Here's how the part is built. I have some questions about the finished solid (model axes, mm). Round coordinates to 2 decimals unless told otherwise and drop trailing zeros. Order: outer loops, then holes, each group sorted by start corner. A loop starts at its lowest first (then second) coordinate and runs counter-clockwise, first axis right, second up. Notation, with made-up numbers: (-3.5, 56.25) -> (25.5, 56.25) arc R21 cw to (25.5, 65.25) -> close; hole circle Ø10 at (66.5, -9). An arc over 180 degrees is marked (long way). Use a Markdown table: item, result. Add a question column.
(1) I want a section at A-A, the plane z = -196. Please give me the cut outline in (x, y) (3 decimals).
(2) I'm going to push flat-ended pins straight in: P1, Ø4.5, axis at y = 4.63, z = -273.28, coming from the +X side; P2, Ø1.6, axis at x = 1, z = -390, coming from the -Y side; P3, Ø1, axis at x = 1.5, z = -354, coming from the -Y side; P4, Ø1, axis at x = 2.5, z = -388.5, coming from the +Y side. Where does each tip first touch, or does it pass through?
(3) If I drill on probe 1 along Z at (x, y) = (1.5, 31); probe 2 along Y at (x, z) = (0.85, -200.5); probe 3 along Y at (x, z) = (0.4, -272.5), over which ranges is the centre line in solid material (lowest first)?
(4) I want a section at C-C, the plane x = 2.25. Give the number of separate pieces and of enclosed holes in the cut face, then the cut area to 3 significant figures.
(5) I want a section at D-D, the plane y = 104.5. Please give me the cut outline in (x, z) (3 decimals), then the cut area to 3 significant figures.
(6) I want a section at B-B, the plane z = -59. Please give me the cut outline in (x, y) (3 decimals), then the cut area to 3 significant figures.
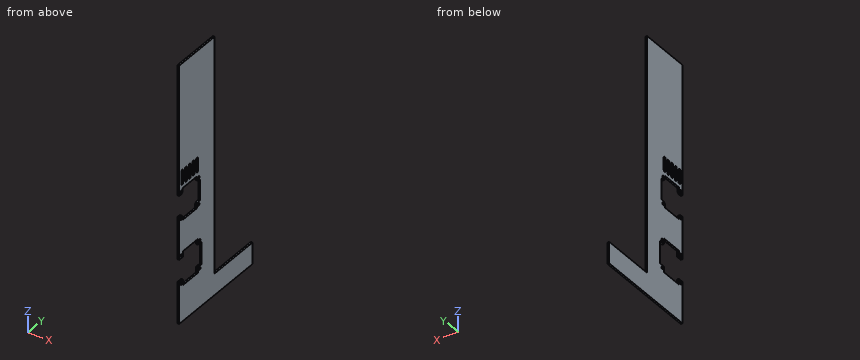
Autodesk Inventor part; units mm, degrees
ref_plane "YZ Plane" through (0, 0, 0) normal (1, 0, 0) x (0, 1, 0)
ref_plane "XZ Plane" through (0, 0, 0) normal (0, 1, 0) x (-1, 0, 0)
ref_plane "XY Plane" through (0, 0, 0) normal (0, 0, 1) x (1, 0, 0)
sketch "Sketch1" plane through (0, 0, 0) normal (1, 0, 0) x (0, 1, 0)
  line L0 (0, 0) -> (95.25, 0)
  line L1 (95.25, 0) -> (95.25, -419.1)
  line L2 (95.25, -457.2) -> (0, -457.2)
  line L3 (0, -457.2) -> (0, 0)
  line L4 (0, -457.2) -> (196.85, -457.2)
  line L5 (196.85, -457.2) -> (196.85, -419.1)
  line L6 (196.85, -419.1) -> (95.25, -419.1)
  line L7 (0, -419.1) -> (0, -457.2)
extrude "Extrusion1" add sketch "Sketch1" along normal blind 3.175
sketch "Sketch2" plane through (0, 0, 0) normal (-1, 0, 0) x (0, 0, 1)
  line L0 (-393.7, 49.9364) -> (-393.7, 10.0076)
  line L1 (-333.756, 10.0076) -> (-333.756, 49.9364)
  line L2 (-343.7636, 59.944) -> (-383.6924, 59.944)
  circle A0 centre (-388.6962, 54.9402) radius 2.159
  circle A1 centre (-338.7598, 54.9402) radius 2.159
  circle A2 centre (-388.6962, 5.0038) radius 2.159
  circle A3 centre (-338.7598, 5.0038) radius 2.159
  line L3 (-383.6924, 59.944) -> (-383.6924, 49.9364)
  line L4 (-383.6924, 49.9364) -> (-393.7, 49.9364)
  line L5 (-343.7636, 59.944) -> (-343.7636, 49.9364)
  line L6 (-343.7636, 49.9364) -> (-333.756, 49.9364)
  line L7 (-383.6924, 0) -> (-383.6924, 10.0076)
  line L8 (-383.6924, 10.0076) -> (-393.7, 10.0076)
  line L9 (-343.7636, 0) -> (-343.7636, 10.0076)
  line L10 (-343.7636, 10.0076) -> (-333.756, 10.0076)
  circle A4 centre (-273.2786, 51.7724) radius 2.54
  circle A5 centre (-273.2786, 4.63) radius 2.54
  circle A6 centre (-226.1362, 51.7724) radius 2.54
  circle A7 centre (-226.1362, 4.63) radius 2.54
  line L11 (-190.9572, 5.646) -> (-212.4456, 5.646)
  line L12 (-212.4456, 10.726) -> (-190.9572, 10.726)
  arc A8 (-190.9572, 5.646) -> (-190.9572, 10.726) centre (-190.9572, 8.186) ccw
  arc A9 (-212.4456, 10.726) -> (-212.4456, 5.646) centre (-212.4456, 8.186) ccw
  line L13 (-190.9572, 15.6282) -> (-212.4456, 15.6282)
  line L14 (-212.4456, 20.7082) -> (-190.9572, 20.7082)
  arc A10 (-190.9572, 15.6282) -> (-190.9572, 20.7082) centre (-190.9572, 18.1682) ccw
  arc A11 (-212.4456, 20.7082) -> (-212.4456, 15.6282) centre (-212.4456, 18.1682) ccw
  line L15 (-190.9572, 25.6104) -> (-212.4456, 25.6104)
  line L16 (-212.4456, 30.6904) -> (-190.9572, 30.6904)
  arc A12 (-190.9572, 25.6104) -> (-190.9572, 30.6904) centre (-190.9572, 28.1504) ccw
  arc A13 (-212.4456, 30.6904) -> (-212.4456, 25.6104) centre (-212.4456, 28.1504) ccw
  line L17 (-190.9572, 35.5926) -> (-212.4456, 35.5926)
  line L18 (-212.4456, 40.6726) -> (-190.9572, 40.6726)
  arc A14 (-190.9572, 35.5926) -> (-190.9572, 40.6726) centre (-190.9572, 38.1326) ccw
  arc A15 (-212.4456, 40.6726) -> (-212.4456, 35.5926) centre (-212.4456, 38.1326) ccw
  line L19 (-190.9572, 45.5748) -> (-212.4456, 45.5748)
  line L20 (-212.4456, 50.6548) -> (-190.9572, 50.6548)
  arc A16 (-190.9572, 45.5748) -> (-190.9572, 50.6548) centre (-190.9572, 48.1148) ccw
  arc A17 (-212.4456, 50.6548) -> (-212.4456, 45.5748) centre (-212.4456, 48.1148) ccw
  line L21 (-457.2, 0) -> (-457.2, 196.85)
  line L22 (-457.2, 0) -> (-393.7, 0)
  line L23 (-383.6924, 0) -> (-343.7636, 0)
  line L24 (-419.1, 95.25) -> (0, 95.25)
  line L25 (-4.8028, 0) -> (-4.8028, 95.25)
  line L26 (-4.8028, 95.25) -> (-457.2, 95.25)
  line L27 (-457.2, 95.25) -> (-457.2, 0)
  line L28 (-267.3803, 56.4007) -> (-232.0345, 56.4007)
  line L29 (-221.5079, 45.8741) -> (-221.5079, 10.5283)
  line L30 (-232.0345, 0) -> (-267.3803, 0)
  line L31 (-277.9086, 10.5283) -> (-277.9086, 45.8741)
  line L32 (-273.2786, 51.7724) -> (-271.5234, 49.9364)
  line L33 (-271.5234, 49.9364) -> (-270.4878, 48.8532)
  arc A18 (-268.6503, 4.5045) -> (-273.4041, 9.2583) centre (-273.2786, 4.63) ccw
  arc A19 (-226.1362, 9.2583) -> (-230.7645, 4.63) centre (-226.1362, 4.63) ccw
  arc A20 (-230.7645, 51.7724) -> (-226.1362, 47.1441) centre (-226.1362, 51.7724) ccw
  arc A21 (-273.2786, 47.1441) -> (-268.6503, 51.7724) centre (-273.2786, 51.7724) ccw
  line L34 (-268.6503, 55.1307) -> (-268.6503, 51.7724)
  line L35 (-273.2786, 47.1441) -> (-276.6386, 47.1441)
  line L36 (-230.7645, 55.1307) -> (-230.7645, 51.7724)
  line L37 (-226.1362, 47.1441) -> (-222.7779, 47.1441)
  line L38 (-221.5079, 0) -> (-230.7645, 0)
  line L39 (-230.7645, 1.27) -> (-230.7645, 4.63)
  line L40 (-226.1362, 9.2583) -> (-222.7779, 9.2583)
  line L41 (-277.9086, 0) -> (-268.6503, 0)
  line L42 (-268.6503, 1.27) -> (-268.6503, 4.7555)
  line L43 (-273.1531, 9.2583) -> (-276.6386, 9.2583)
  arc A22 (-277.9086, 10.5283) -> (-276.6386, 9.2583) centre (-276.6386, 10.5283) ccw
  arc A23 (-267.3803, 56.4007) -> (-268.6503, 55.1307) centre (-267.3803, 55.1307) ccw
  arc A24 (-276.6386, 47.1441) -> (-277.9086, 45.8741) centre (-276.6386, 45.8741) ccw
  arc A25 (-230.7645, 55.1307) -> (-232.0345, 56.4007) centre (-232.0345, 55.1307) ccw
  arc A26 (-221.5079, 45.8741) -> (-222.7779, 47.1441) centre (-222.7779, 45.8741) ccw
  arc A27 (-222.7779, 9.2583) -> (-221.5079, 10.5283) centre (-222.7779, 10.5283) ccw
  line L44 (-277.9086, 56.4007) -> (-277.7032, 56.4007)
  line L45 (-268.6503, 4.5045) -> (-268.6503, 0)
  line L46 (0, 0) -> (-457.2, 0)
  line L47 (-230.7645, 4.63) -> (-230.7645, 0)
  line L48 (-268.6503, 0) -> (-230.7645, 0)
  dimension "d50" = 1.4986
  dimension "d52" = 1.27
extrude "Extrusion2" cut sketch "Sketch2" against normal blind 25.4 contours L4 L3 L2 L5 L6 L1 L10 L9 L23 L7 L8 L0 | L45 L42 A18 L43 A22 L31 A24 L35 A21 L34 A23 L28 A25 L36 A20 L37 A26 L29 A27 L40 A19 L39 L47 L46 L30 | A0 | A1 | A2 | A3 | A4 | A5 | A6 | A7 | L11 A9 L12 A8 | L13 A11 L14 A10 | L15 A13 L16 A12 | L17 A15 L18 A14 | L19 A17 L20 A16
sketch "Sketch6" plane through (3.175, 0, 0) normal (1, 0, 0) x (0, 0, -1)
  point P0 (0, 0)
properties part number "220228 Left Side with brace"
Taken from the geometry:
| question | item | result |
|---|---|---|
| 1 | outline | (0, 0) -> (3.175, 0) -> (3.175, 5.646) -> (0, 5.646) -> close; (0, 10.726) -> (3.175, 10.726) -> (3.175, 15.628) -> (0, 15.628) -> close; (0, 20.708) -> (3.175, 20.708) -> (3.175, 25.61) -> (0, 25.61) -> close; (0, 30.69) -> (3.175, 30.69) -> (3.175, 35.593) -> (0, 35.593) -> close; (0, 40.673) -> (3.175, 40.673) -> (3.175, 45.575) -> (0, 45.575) -> close; (0, 50.655) -> (3.175, 50.655) -> (3.175, 95.25) -> (0, 95.25) -> close |
| 2 | P1 | passes through |
| 2 | P2 | stops at y = 0 |
| 2 | P3 | stops at y = 59.94 |
| 2 | P4 | stops at y = 95.25 |
| 3 | probe 1 | z = -457.2 to -393.7, -333.76 to -277.91, -221.51 to 0 |
| 3 | probe 2 | y = 0 to 5.65, 10.73 to 15.63, 20.71 to 25.61, 30.69 to 35.59, 40.67 to 45.57, 50.65 to 95.25 |
| 3 | probe 3 | y = 0 to 2.21, 7.05 to 9.19, 47.21 to 49.35, 54.19 to 95.25 |
| 4 | separate pieces | 1 |
| 4 | enclosed holes | 13 |
| 4 | area | 40,600 mm2 |
| 5 | outline | (0, -457.2) -> (3.175, -457.2) -> (3.175, -419.1) -> (0, -419.1) -> close |
| 5 | area | 121 mm2 |
| 6 | outline | (0, 0) -> (3.175, 0) -> (3.175, 95.25) -> (0, 95.25) -> close |
| 6 | area | 302 mm2 |
